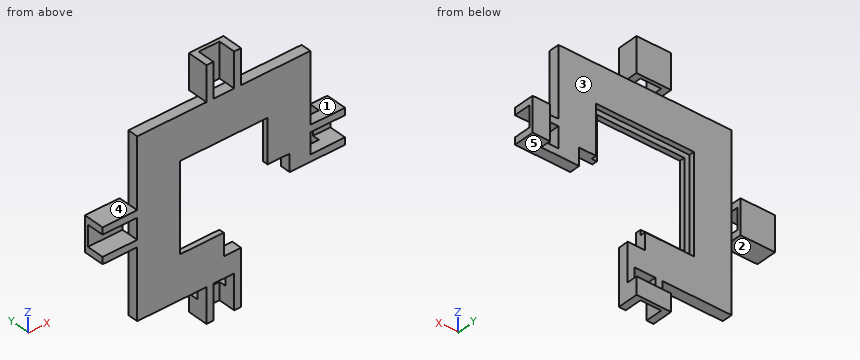
from build123d import *

# Parameters (mm, degrees)
BOSS_EXTRUDE10_DEPTH = 12
SKETCH6_W            = 100
SKETCH6_H            = 100
CUT_EXTRUDE1_DEPTH   = 6
SKETCH7_W            = 20
SKETCH7_H            = 12
SKETCH7_W_2          = 12
SKETCH7_H_2          = 20
CUT_EXTRUDE2_DEPTH   = 10
SKETCH8_W            = 56.5
SKETCH8_H            = 56.5
CUT_EXTRUDE3_DEPTH   = 3
SKETCH10_W           = 20
SKETCH10_H           = 10
SKETCH10_W_2         = 10
SKETCH10_H_2         = 20
CUT_EXTRUDE6_DEPTH   = 6
SKETCH11_W           = 10
SKETCH11_H           = 12.75
SKETCH11_W_2         = 12.75
SKETCH11_H_2         = 10
CUT_EXTRUDE7_DEPTH   = 100.176610146


with BuildPart() as part:
    # Sketch1 → Boss-Extrude10 (new body)
    with BuildSketch(Plane(origin=(0, 0, 0), x_dir=(1, 0, 0), z_dir=(0, 1, 0))):
        Polygon((-50, 50), (-10, 50), (-10, 70), (10, 70), (10, 25.25), (-25.25, 25.25), (-25.25, -25.25), (25.25, -25.25), (25.25, 10), (70, 10), (70, -10), (50, -10), (50, -50), (10, -50), (10, -70), (-10, -70), (-10, -50), (-50, -50), (-50, -10), (-70, -10), (-70, 10), (-50, 10), align=None)
    extrude(amount=BOSS_EXTRUDE10_DEPTH)

    # Sketch6 → Cut-Extrude1 (cut)
    with BuildSketch(Plane(origin=(0, 12, 0), x_dir=(1, 0, 0), z_dir=(0, 1, 0))):
        Rectangle(SKETCH6_W, SKETCH6_H)
    extrude(amount=-CUT_EXTRUDE1_DEPTH, mode=Mode.SUBTRACT)

    # Sketch7 → Cut-Extrude2 (cut)
    with BuildSketch(Plane(origin=(0, 0, 0), x_dir=(-1, 0, 0), z_dir=(0, -1, 0))):
        with Locations((60, 0)):
            Rectangle(SKETCH7_W, SKETCH7_H)
        with Locations((0, -60)):
            Rectangle(SKETCH7_W_2, SKETCH7_H_2)
        with Locations((-60, 0)):
            Rectangle(SKETCH7_W, SKETCH7_H)
        with Locations((0, 60)):
            Rectangle(SKETCH7_W_2, SKETCH7_H_2)
    extrude(amount=-CUT_EXTRUDE2_DEPTH, mode=Mode.SUBTRACT)

    # Sketch8 → Cut-Extrude3 (cut)
    with BuildSketch(Plane(origin=(0, 6, 0), x_dir=(1, 0, 0), z_dir=(0, 1, 0))):
        Rectangle(SKETCH8_W, SKETCH8_H)
    extrude(amount=-CUT_EXTRUDE3_DEPTH, mode=Mode.SUBTRACT)

    # Sketch10 → Cut-Extrude6 (cut)
    with BuildSketch(Plane(origin=(0, 12, 0), x_dir=(1, 0, 0), z_dir=(0, 1, 0))):
        with Locations((0, 55)):
            Rectangle(SKETCH10_W, SKETCH10_H)
        with Locations((55, 0)):
            Rectangle(SKETCH10_W_2, SKETCH10_H_2)
    extrude(amount=-CUT_EXTRUDE6_DEPTH, mode=Mode.SUBTRACT)

    # Sketch11 → Cut-Extrude7 (cut, through all)
    with BuildSketch(Plane(origin=(0, 6, 0), x_dir=(1, 0, 0), z_dir=(0, 1, 0))):
        with Locations((5, 31.625)):
            Rectangle(SKETCH11_W, SKETCH11_H)
        with Locations((31.625, 5)):
            Rectangle(SKETCH11_W_2, SKETCH11_H_2)
    extrude(amount=-CUT_EXTRUDE7_DEPTH, mode=Mode.SUBTRACT)


solid = part.part
Geometry: final body of the model. Coordinates: model frame, mm. Face numbers are marked on the shaded views. A direction names the side the tool comes from. Coordinates: 2 decimals unless noted, no trailing zeros. Order: outer loops, then holes, each group sorted by start corner. A loop starts at its lowest first (then second) coordinate and runs counter-clockwise, first axis right, second up.
1) Ray query, probe 1 along X at (y, z) = (9, 55); probe 2 along Z at (x, y) = (-7, 2); probe 3 along X at (y, z) = (0.5, 1.5). Return the intervals inside material, ascending.
Result sheet:
probe 1: x = -10 to -6, 6 to 10
probe 2: z = -70 to -25.25, 25.25 to 70
probe 3: x = -50 to -25.25, 25.25 to 50
2) Section D-D (x = -52). Return loops of the section in (y, z), then the cut area to 3 significant figures.
Result sheet:
outline: (0, -10) - (12, -10) - (12, 10) - (0, 10) - (0, 6) - (10, 6) - (10, -6) - (0, -6) - close
area: 120 mm2
3) Section B-B (z = -8). Return loops of the section in (x, y).
Result sheet:
outline: (-70, 0) - (-25.25, 0) - (-25.25, 3) - (-28.25, 3) - (-28.25, 6) - (-50, 6) - (-50, 12) - (-70, 12) - close; (38, 0) - (70, 0) - (70, 12) - (60, 12) - (60, 6) - (38, 6) - close
4) Section A-A (x = 53). Return loops of the section in (y, z).
Result sheet:
outline: (0, -10) - (6, -10) - (6, -6) - (0, -6) - close; (0, 6) - (6, 6) - (6, 10) - (0, 10) - close
5) Section C-C (z = 56). Return loops of the section in (x, y).
Result sheet:
outline: (-10, 0) - (-6, 0) - (-6, 10) - (6, 10) - (6, 0) - (10, 0) - (10, 12) - (-10, 12) - close
6) Set-up query: the marked faces 1, 2, 3, 4 and 5. Return all of +Z, -Z, +X, -X, +Y, -Y with unobstructed straight access to the full face (end or side cutting, diameter ignored); none if empty.
Result sheet:
face 1: +Z, +X, +Y, -Y
face 2: -Z, -X, +Y, -Y
face 3: +Y
face 4: +Z, -X, +Y, -Y
face 5: -Z, +X, +Y, -Y
7) First-contact query: P1, Ø3, axis at y = 5, z = -39, coming from the +X side; P2, Ø1, axis at x = -2, y = 2.5, coming from the +Z side; P3, Ø1.5, axis at x = -49.5, z = 6, coming from the +Y side; P4, Ø5, axis at y = 4.5, z = 36.5, coming from the -X side. Flat tips, straight axial feed; report the tip coordinate or a pass-through.
Result sheet:
P1: stops at x = 10
P2: stops at z = 50
P3: stops at y = 12
P4: stops at x = -50
